from build123d import *

# Parameters (mm, degrees)
SALIENTE_EXTRUIR3_DEPTH = 34
CROQUIS6_R              = 19.75
CORTAR_EXTRUIR2_DEPTH   = 68.683085036
VACIADO3_T              = -2
CROQUIS5_R              = 1.5
CORTAR_EXTRUIR3_DEPTH   = 10
REDONDEO1_R             = 5
REDONDEO3_R             = 5
CROQUIS10_R             = 4
CORTAR_EXTRUIR7_DEPTH   = 67.068146637
REDONDEO4_R             = 4


with BuildPart() as part:
    # Croquis4 → Saliente-Extruir3 (new body)
    with BuildSketch(Plane(origin=(0, 0, 0), x_dir=(0, 0, -1), z_dir=(1, 0, 0))):
        Polygon((0, 0), (55, 0), (0, 20), align=None)
    extrude(amount=SALIENTE_EXTRUIR3_DEPTH)

    # Croquis6 → Cortar-Extruir2 (cut, through all)
    with BuildSketch(Plane.XY):
        with Locations((17, -17)):
            Circle(CROQUIS6_R)
    extrude(amount=-CORTAR_EXTRUIR2_DEPTH, mode=Mode.SUBTRACT)

    # Vaciado3
    vaciado3_openings = [part.faces().sort_by_distance(p)[0] for p in [
        (17, 10.517691614, -26.076348062),
    ]]
    offset(amount=VACIADO3_T, openings=vaciado3_openings, kind=Kind.INTERSECTION)

    # Croquis5 → Cortar-Extruir3 (cut)
    with BuildSketch(Plane.XY):
        with Locations((4.5, 15)):
            Circle(CROQUIS5_R)
        with Locations((29.5, 15)):
            Circle(CROQUIS5_R)
        with Locations((29.5, 5)):
            Circle(CROQUIS5_R)
        with Locations((4.5, 5)):
            Circle(CROQUIS5_R)
    extrude(amount=-CORTAR_EXTRUIR3_DEPTH, mode=Mode.SUBTRACT)

    # Redondeo1
    redondeo1_edges = [part.edges().sort_by_distance(p)[0] for p in [
        (27.052984631, 0, -27.5),
        (6.947015369, 0, -27.5),
    ]]
    fillet(redondeo1_edges, radius=REDONDEO1_R)

    # Redondeo3
    redondeo3_edges = [part.edges().sort_by_distance(p)[0] for p in [
        (6.41404232, 2, -25.750000004),
        (27.58595768, 2, -25.75),
    ]]
    fillet(redondeo3_edges, radius=REDONDEO3_R)

    # Croquis10 → Cortar-Extruir7 (cut, through all)
    with BuildSketch(Plane(origin=(0, 0, -2), x_dir=(-1, 0, 0), z_dir=(0, 0, -1))):
        with Locations((-29.5, 15)):
            Circle(CROQUIS10_R)
        with Locations((-4.5, 15)):
            Circle(CROQUIS10_R)
        with Locations((-4.5, 5)):
            Circle(CROQUIS10_R)
        with Locations((-29.5, 5)):
            Circle(CROQUIS10_R)
    extrude(amount=CORTAR_EXTRUIR7_DEPTH, mode=Mode.SUBTRACT)

    # Redondeo4
    redondeo4_edges = [part.edges().sort_by_distance(p)[0] for p in [
        (2, 8.122498999, -17.331563876),
        (2, 11.877501001, -12.168436124),
        (32, 8.122498999, -17.331563876),
        (32, 11.877501001, -12.168436124),
    ]]
    fillet(redondeo4_edges, radius=REDONDEO4_R)


solid = part.part
Part model, mm, in its own coordinate system. A direction names the side the tool comes from. Give positions to 0.01 mm unless a question says otherwise; leave off trailing zeros. Order: outer loops, then holes, each group sorted by start corner. A loop starts at its lowest first (then second) coordinate and runs counter-clockwise, first axis right, second up. Notation, with made-up numbers: (48.25, 7.5) -> (65.25, 7.5) arc R33 ccw to (65.25, 41.5) -> close; hole circle Ø4 at (-9, 43). An arc over 180 degrees is marked (long way). Use one line per item in the form item = value.
(1) Saw through at A-A (x = 4.5). Write the cut outline in (y, z), then the cut area to 3 significant figures.
Solution:
outline = (0, -55) -> (1, -52.25) -> (1, -2) -> (3.5, -2) -> (3.5, 0) -> (0, 0) -> close; (6.5, -2) -> (13.5, -2) -> (13.5, 0) -> (6.5, 0) -> close; (16.5, -2) -> (19.27, -2) -> (20, 0) -> (16.5, 0) -> close
area = 78.9 mm²
(2) Saw through at B-B (y = 15). Write the cut outline in (x, z).
Solution:
outline = (0, -13.75) -> (0.5, -13.75) -> (0.5, -2) -> (3, -2) -> (3, 0) -> (0, 0) -> close; (6, -2) -> (28, -2) -> (28, 0) -> (6, 0) -> close; (31, -2) -> (33.5, -2) -> (33.5, -13.75) -> (34, -13.75) -> (34, 0) -> (31, 0) -> close
(3) Drill centre lines: line 1 (Y direction, x = 29.5, z = -1.15); line 2 (Y direction, x = 4.5, z = -0.65); line 3 (Z direction, x = 19.5, y = 17.5). Where is each one in solid material? Low to high. Write a range as from..to.
Solution:
line_1 = 0..3.5, 6.5..13.5, 16.5..19.58
line_2 = 0..3.5, 6.5..13.5, 16.5..19.76
line_3 = -2..0
(4) Flat gauge pins, fed straight in: P1, Ø5, axis at x = 18, z = -48.5, coming from the +Y side; P2, Ø5, axis at x = 29.5, y = 5, coming from the -Z side; P3, Ø4, axis at x = 29.5, y = 15, coming from the +Z side; P4, Ø5, axis at x = 23, z = -17, coming from the +Y side. Where does each tip first touch, or does it go through?
Solution:
P1 = 3.27
P2 = -2
P3 = 0
P4 = 4.47
(5) Saw through at D-D (z = -18). Write the cut outline in (x, y).
Solution:
outline = (0, 0) -> (5.66, 0) arc R5 ccw to (7.95, 0.56) arc R19.75 cw to (26.05, 0.56) arc R5 ccw to (28.34, 0) -> (34, 0) -> (34, 13.45) -> (33.19, 13.45) arc R4 cw to (32.75, 12.67) arc R4 ccw to (32, 10.34) -> (32, 9.66) arc R4 ccw to (32.75, 7.33) arc R4 cw (long way) to (26.23, 2.69) arc R21.75 ccw to (7.77, 2.69) arc R4 cw (long way) to (1.25, 7.33) arc R4 ccw to (2, 9.66) -> (2, 10.34) arc R4 ccw to (1.25, 12.67) arc R4 cw to (0.81, 13.45) -> (0, 13.45) -> close
(6) Tool access for faces 4 (the face through (32, 18.5, -2.9)), 5 (the face through (6.824, 0.137, -27.115)), 6 (the face through (5.886, 4.425, -0.986)): list every direction of +Z, -Z, +X, -X, +Y, -Y with a clear straight run to the whole face (end or side of a thin tool).
Solution:
face_4 = -Z, +Y
face_5 = +Z, -Z, -Y
face_6 = +Z, -Z
(7) Pull direction Y, two halves, no side cores. Call faces 1 (the face through (31, 0, -27)), 2 (the face through (0, 6, -15)), 3 (the face through (28, 5, -1)): +Y half, -Y half, draft (parallel to the pull), parting line (faces both ways), or undercut.
Solution:
face_1 = -Y half
face_2 = draft
face_3 = undercut
(8) Saw through at C-C (z = -49). Write the cut outline in (x, y), then the cut area to 3 significant figures.
Solution:
outline = (0, 0) -> (5.66, 0) arc R5 ccw to (7.95, 0.56) arc R19.75 cw to (12.3, 2.18) -> (7.34, 2.18) arc R4 cw to (1.66, 2.18) -> (0, 2.18) -> close; (21.7, 2.18) arc R19.75 cw to (26.05, 0.56) arc R5 ccw to (28.34, 0) -> (34, 0) -> (34, 2.18) -> (32.34, 2.18) arc R4 cw to (26.66, 2.18) -> close
area = 30.8 mm²
